Part model, mm, in its own coordinate system. A direction names the side the tool comes from. Round coordinates to 2 decimals unless told otherwise and drop trailing zeros. Loops run counter-clockwise (first coordinate to the right, second up) from the corner with the lowest first, then second, coordinate; pieces in that order, holes last.
(1) Mould opens along Y. For faces 3 (the face through (-36.596, -79.415, 9.86)), 4 (the face through (-1, -17, 20)), 5 (the face through (-27.81, -15.83, 9.86)) say: +Y half, -Y half, draft (parallel to the pull), parting line (faces both ways), or undercut.
(2) Cut at C-C on x = -56. List the corners of the cut face in (y, z).
(3) Cut at B-B on y = 0. List the corners of the cut face in (x, z).
(4) Cut at A-A on x = 0. List the corners of the cut face in (y, z).
(5) Tool access for faces 1 (the face through (15.72, -21.23, 9.86)), 2 (the face through (-5.21, 39.66, 12.08)): list every direction of +Z, -Z, +X, -X, +Y, -Y with a clear straight run to the whole face (end or side of a thin tool).
(6) Flat gauge pins, fed straight in: pin 1 (2 mm diameter, centred on y = -70, z = 17, fed in from +X); pin 2 (3 mm diameter, centred on x = 47, z = 3.5, fed in from -Y); pin 3 (25 mm diameter, centred on x = 10.5, y = -31, fed in from +Z). Where does each tip first touch, or does it go through?
(7) Probe probe 1 along Y at (x, z) = (27, 8.75); probe 2 along X at (y, z) = (14.5, 1.5); probe 3 along X at (y, z) = (3.5, 12.25). List the from-to ranges inside material, lowest first.
(8) Cut at D-D on z = 22.25. List the corners of the cut face in (x, y), then the cut area to 3 significant figures.
from build123d import *

# Parameters (mm, degrees)
SKETCH3_R             = 40
SKETCH3_R_2           = 16
BOSS_EXTRUDE1_DEPTH   = 20
BOSS_EXTRUDE1_2_DEPTH = 20
BOSS_EXTRUDE1_3_DEPTH = 20
BOSS_EXTRUDE2_DEPTH   = 10
SKETCH3_4_R           = 20
SKETCH3_4_R_2         = 15
SKETCH3_4_R_3         = 21
BOSS_EXTRUDE3_DEPTH   = 30


with BuildPart() as part:
    # Sketch3 → Boss-Extrude1 (new body)
    with BuildSketch(Plane.XY):
        Circle(SKETCH3_R)
        Circle(SKETCH3_R_2, mode=Mode.SUBTRACT)
        with BuildLine():
            ThreePointArc((-13.331456111, -29.090759323), (0, -32), (13.331456111, -29.090759323))
            Line((13.331456111, -29.090759323), (7.794228634, -19.5))
            ThreePointArc((7.794228634, -19.5), (0, -21), (-7.794228634, -19.5))
            Line((-7.794228634, -19.5), (-13.331456111, -29.090759323))
        make_face(mode=Mode.SUBTRACT)
        with BuildLine():
            ThreePointArc((18.527608533, -26.090759323), (27.712812921, -16), (31.859064644, -3))
            Line((31.859064644, -3), (20.784609691, -3))
            ThreePointArc((20.784609691, -3), (18.186533479, -10.5), (12.990381057, -16.5))
            Line((12.990381057, -16.5), (18.527608533, -26.090759323))
        make_face(mode=Mode.SUBTRACT)
        with BuildLine():
            ThreePointArc((31.859064644, 3), (27.712812921, 16), (18.527608533, 26.090759323))
            Line((18.527608533, 26.090759323), (12.990381057, 16.5))
            ThreePointArc((12.990381057, 16.5), (18.186533479, 10.5), (20.784609691, 3))
            Line((20.784609691, 3), (31.859064644, 3))
        make_face(mode=Mode.SUBTRACT)
        with BuildLine():
            ThreePointArc((13.331456111, 29.090759323), (0, 32), (-13.331456111, 29.090759323))
            Line((-13.331456111, 29.090759323), (-7.794228634, 19.5))
            ThreePointArc((-7.794228634, 19.5), (0, 21), (7.794228634, 19.5))
            Line((7.794228634, 19.5), (13.331456111, 29.090759323))
        make_face(mode=Mode.SUBTRACT)
        with BuildLine():
            Line((-12.990381057, 16.5), (-18.527608533, 26.090759323))
            ThreePointArc((-18.527608533, 26.090759323), (-27.712812921, 16), (-31.859064644, 3))
            Line((-31.859064644, 3), (-20.784609691, 3))
            ThreePointArc((-20.784609691, 3), (-18.186533479, 10.5), (-12.990381057, 16.5))
        make_face(mode=Mode.SUBTRACT)
        with BuildLine():
            Line((-20.784609691, -3), (-31.859064644, -3))
            ThreePointArc((-31.859064644, -3), (-27.712812921, -16), (-18.527608533, -26.090759323))
            Line((-18.527608533, -26.090759323), (-12.990381057, -16.5))
            ThreePointArc((-12.990381057, -16.5), (-18.186533479, -10.5), (-20.784609691, -3))
        make_face(mode=Mode.SUBTRACT)
    extrude(amount=BOSS_EXTRUDE1_DEPTH)



with BuildPart() as body_2:
    # Sketch3 → Boss-Extrude1 2 (new body)
    with BuildSketch(Plane.XY):
        with BuildLine():
            Line((-66.324952937, -70.02485881), (-6.023764702, -89.071294105))
            ThreePointArc((-6.023764702, -89.071294105), (-19.833394958, -72.576129737), (-10.695968955, -53.100406866))
            ThreePointArc((-10.695968955, -53.100406866), (-27.903629702, -55.111072059), (-40.22513893, -42.932124106))
            ThreePointArc((-40.22513893, -42.932124106), (-39.308551495, -46.413363865), (-39, -50))
            ThreePointArc((-39, -50), (-47.586781474, -66.938477081), (-66.324952937, -70.02485881))
        make_face()
    extrude(amount=BOSS_EXTRUDE1_2_DEPTH)


with BuildPart() as body_3:
    # Sketch3 → Boss-Extrude1 3 (new body)
    with BuildSketch(Plane.XY):
        with BuildLine():
            Line((6.023764702, -89.071294105), (66.324952937, -70.02485881))
            ThreePointArc((66.324952937, -70.02485881), (44.876208292, -64.569520389), (40.22513893, -42.932124106))
            ThreePointArc((40.22513893, -42.932124106), (27.903629702, -55.111072059), (10.695968955, -53.100406866))
            ThreePointArc((10.695968955, -53.100406866), (17.520265111, -60.354259466), (20, -70))
            ThreePointArc((20, -70), (16.131882935, -81.822112882), (6.023764702, -89.071294105))
        make_face()
    extrude(amount=BOSS_EXTRUDE1_3_DEPTH)


with BuildPart() as part_1:
    add(part.part)

    add(body_2.part)  # Boss-Extrude2 merges body 2

    add(body_3.part)  # Boss-Extrude2 merges body 3
    # Sketch3_3 → Boss-Extrude2 (add)
    with BuildSketch(Plane.XY):
        with BuildLine():
            ThreePointArc((10.695968955, -53.100406866), (27.903629702, -55.111072059), (40.22513893, -42.932124106))
            ThreePointArc((40.22513893, -42.932124106), (47.76318349, -32.933649432), (59.651863383, -29.002885891))
            ThreePointArc((59.651863383, -29.002885891), (44.262528341, -22.168588856), (39.546869801, -6.003756239))
            ThreePointArc((39.546869801, -6.003756239), (0, -40), (-39.546869801, -6.003756239))
            ThreePointArc((-39.546869801, -6.003756239), (-44.262528341, -22.168588856), (-59.651863383, -29.002885891))
            ThreePointArc((-59.651863383, -29.002885891), (-47.76318349, -32.933649432), (-40.22513893, -42.932124106))
            ThreePointArc((-40.22513893, -42.932124106), (-27.903629702, -55.111072059), (-10.695968955, -53.100406866))
            ThreePointArc((-10.695968955, -53.100406866), (0, -50), (10.695968955, -53.100406866))
        make_face()
    extrude(amount=BOSS_EXTRUDE2_DEPTH)

    # Sketch3_4 → Boss-Extrude3 (add)
    # profile 1 of 3: a face of its own
    with BuildSketch(Plane.XY):
        with Locations(Location((0, -70, 0), (0, 0, 122.33024367))):
            Circle(SKETCH3_4_R)
        with Locations((0, -70)):
            Circle(SKETCH3_4_R_2, mode=Mode.SUBTRACT)
    # profile 2 of 3: a face of its own
    with BuildSketch(Plane.XY):
        with Locations(Location((-60, -50, 0), (0, 0, 252.471014746))):
            Circle(SKETCH3_4_R_3)
        with Locations((-60, -50)):
            Circle(SKETCH3_4_R_2, mode=Mode.SUBTRACT)
    # profile 3 of 3: a face of its own
    with BuildSketch(Plane.XY):
        with Locations(Location((60, -50, 0), (0, 0, 160.332235519))):
            Circle(SKETCH3_4_R_3)
        with Locations((60, -50)):
            Circle(SKETCH3_4_R_2, mode=Mode.SUBTRACT)
    extrude(amount=BOSS_EXTRUDE3_DEPTH)


solid = part_1.part
Final values:
1. face 3: -Y half
1. face 4: draft
1. face 5: undercut
2. outline: (-73.29, 0) - (-64.46, 0) - (-64.46, 30) - (-70.62, 30) - (-70.62, 20) - (-73.29, 20) - close; (-35.54, 0) - (-28.73, 0) - (-28.73, 10) - (-29.38, 10) - (-29.38, 30) - (-35.54, 30) - close
3. outline: (-40, 0) - (-16, 0) - (-16, 20) - (-40, 20) - close; (16, 0) - (40, 0) - (40, 20) - (16, 20) - close
4. outline: (-90, 0) - (-85, 0) - (-85, 30) - (-90, 30) - close; (-55, 0) - (-32, 0) - (-32, 20) - (-40, 20) - (-40, 10) - (-50, 10) - (-50, 30) - (-55, 30) - close; (-21, 0) - (-16, 0) - (-16, 20) - (-21, 20) - close; (16, 0) - (21, 0) - (21, 20) - (16, 20) - close; (32, 0) - (40, 0) - (40, 20) - (32, 20) - close
5. face 1: +Z, -Z
5. face 2: +Z
6. pin 1: stops at x = 68.94
6. pin 2: stops at y = -76.6
6. pin 3: stops at z = 20
7. probe 1: y = -82.45 to -17.18, -3 to 3, 17.18 to 29.51
7. probe 2: x = -37.28 to -28.53, -15.19 to -6.76, 6.76 to 15.19, 28.53 to 37.28
7. probe 3: x = -39.85 to -31.81, -20.71 to -15.61, 15.61 to 20.71, 31.81 to 39.85
8. outline: circle Ø42 at (-60, -50); circle Ø40 at (0, -70); circle Ø42 at (60, -50); hole circle Ø30 at (-60, -50); hole circle Ø30 at (0, -70); hole circle Ø30 at (60, -50)
8. area: 1,910 mm2
